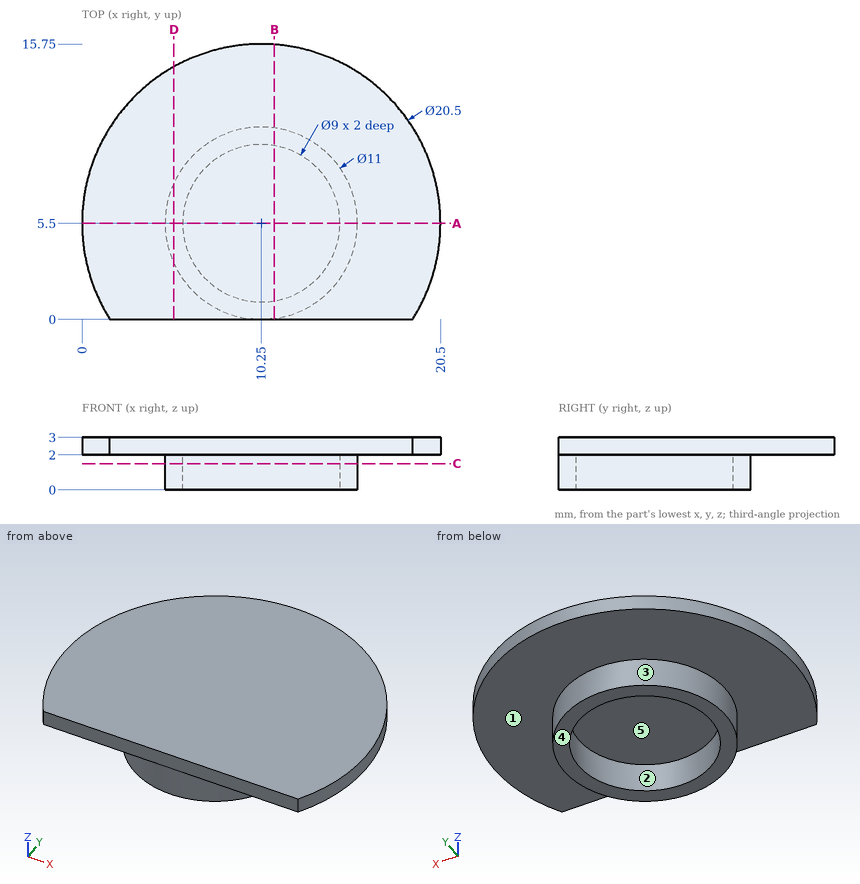
Print and shaded views of the part. All mm, measured from the part's lowest x, y and z. A direction names the side the tool comes from. Coordinates: 2 decimals unless noted, no trailing zeros. Write each loop counter-clockwise with the first axis right and the second up, starting at its lowest first coordinate (ties: lowest second). Pieces come first, ordered by that corner, then holes.
(1) Cut at C-C, the plane z = 1.5. List the corners of the cut face in (x, y).
(2) Cut at B-B, the plane x = 11. List the corners of the cut face in (y, z).
(3) Two-plate mould, pull along X, no slides. Class the marked faces 1, 2 and 3: +X half, -X half, draft (parallel to the pull), parting line (faces both ways), or undercut.
(4) Cut at D-D, the plane x = 5.25. List the corners of the cut face in (y, z).
(5) Flat gauge pins, fed straight in: pin 1 (1.5 mm diameter, centred on x = 14.5, y = 12.5, fed in from -Z); pin 2 (1.5 mm diameter, centred on y = 7.5, z = 2, fed in from +X). Where does each tip first touch, or does it go through?
(6) Cut at A-A, the plane y = 5.5. List the corners of the cut face in (x, z).
(7) Drill centre lines: probe 1 along Y at (x, z) = (10.25, 0.85); probe 2 along Z at (x, y) = (10.75, 13.75); probe 3 along X at (y, z) = (6.25, 0.85). Where is each one in solid material? Low to high.
(8) 3-axis set-ups, long thin cutter, end or side, ignore diameter. For the marked faces 4 and 5: which of +Z, -Z, +X, -X, +Y, -Y reach the whole face in a straight line?
Geometry says:
1. outline: circle Ø11 at (10.25, 5.5); hole circle Ø9 at (10.25, 5.5)
2. outline: (0, 2) - (0.05, 2) - (0.05, 0) - (1.06, 0) - (1.06, 2) - (9.94, 2) - (9.94, 0) - (10.95, 0) - (10.95, 2) - (15.72, 2) - (15.72, 3) - (0, 3) - close
3. face 1: draft
3. face 2: undercut
3. face 3: parting line
4. outline: (0, 2) - (3.21, 2) - (3.21, 0) - (7.79, 0) - (7.79, 2) - (14.45, 2) - (14.45, 3) - (0, 3) - close
5. pin 1: stops at z = 2
5. pin 2: stops at x = 20.42
6. outline: (0, 2) - (4.75, 2) - (4.75, 0) - (5.75, 0) - (5.75, 2) - (14.75, 2) - (14.75, 0) - (15.75, 0) - (15.75, 2) - (20.5, 2) - (20.5, 3) - (0, 3) - close
7. probe 1: y = 0 to 1, 10 to 11
7. probe 2: z = 2 to 3
7. probe 3: x = 4.8 to 5.81, 14.69 to 15.7
8. face 4: -Z, +X, -X, +Y, -Y
8. face 5: -Z
